For this review, take the finished solid that the model builds, in its own axes (mm). Face numbers are marked on the shaded views. A direction names the side the tool comes from. Round coordinates to 2 decimals unless told otherwise and drop trailing zeros. Order: outer loops, then holes, each group sorted by start corner. A loop starts at its lowest first (then second) coordinate and runs counter-clockwise, first axis right, second up. Notation, with made-up numbers: M 53.5,75 L 85.5,75 A28 cw 85.5,111 Z; hole C 76.25,66 d9. An arc over 180 degrees is marked long. Put each result on its own line as item: value.
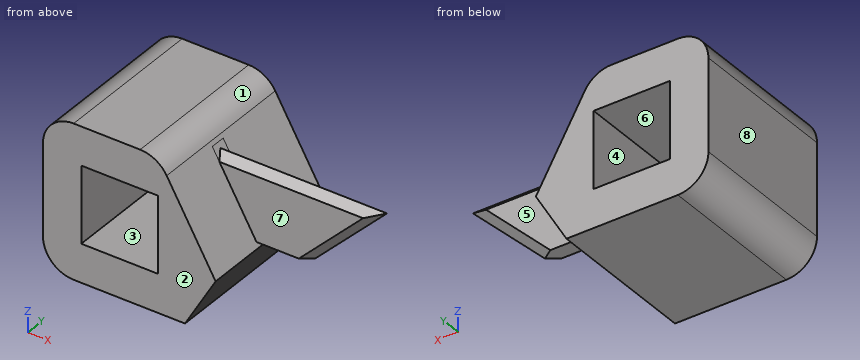
from build123d import *

# Parameters (mm, degrees)
F0_W        = 12.7
F0_H        = 12.7
F1_DEPTH    = 25.4
F4_DEPTH    = 2.54
F5_R        = 5.08
F6_SIZE     = 10.16
F7_T4_DEPTH = 40.3682325584
F7_T9_DEPTH = 40.3682325584
F8_T1_DEPTH = 25.5381499465


# Not quite as in the source:
# - a fillet or chamfer that OpenCascade refuses, or shapes differently, is made with other operations: its cross-section is extruded or revolved along the edge and cut away or added
# - a feature names something its author has since deleted; it is built from what else it names


with BuildPart() as f1:
    # F0 (on Front) → F1 (new body)
    with BuildSketch(Plane.XZ):
        Polygon((19.05, 25.4), (0, 25.4), (0, 0), (33.7146968374, 0), align=None)
        with Locations((12.7, 12.7)):
            Rectangle(F0_W, F0_H, mode=Mode.SUBTRACT)
    extrude(amount=F1_DEPTH)

    # F3 (on mid) → F4 (join)
    with BuildSketch(Plane.XZ.offset(12.7)):
        Polygon((50.8, 22.225), (20.8830871047, 22.225), (28.2154355234, 9.525), (38.1, 9.525), align=None)
    extrude(amount=F4_DEPTH)

    # F5
    f5_edges = [f1.edges().sort_by_distance(p)[0] for p in [
        (0, -12.7, 0),
        (0, -12.7, 25.4),
        (19.05, -12.7, 25.4),
    ]]
    fillet(f5_edges, radius=F5_R)

    # F6
    f6_edges = [f1.edges().sort_by_distance(p)[0] for p in [
        (33.714697, -12.7, 0),
    ]]
    chamfer(f6_edges, length=F6_SIZE)

    # F7: chamfer of 2.032 on 2 edges, made by hand


with BuildPart() as f7_tool2:
    # F7_s3 → F7_t4 (new body)
    with BuildSketch(Plane.YZ.offset(56.0256598315)):
        Polygon((-14.732, 22.225), (-12.7, 20.193), (-12.7, 22.225), align=None)
    extrude(amount=-F7_T4_DEPTH)

    split(bisect_by=Plane(origin=(25.2860226281, 0, 14.598891971), x_dir=(0, 1, 0), z_dir=(0.8660254038, 0, 0.5)), keep=Keep.TOP)


with BuildPart() as f1_1:
    add(f1.part)

    # F7_t1: cut F7_tool2
    add(f7_tool2.part, mode=Mode.SUBTRACT)


with BuildPart() as f7_tool7:
    # F7_s8 → F7_t9 (new body)
    with BuildSketch(Plane.YZ.offset(56.0256598315)):
        Polygon((-15.24, 20.193), (-13.208, 22.225), (-15.24, 22.225), align=None)
    extrude(amount=-F7_T9_DEPTH)

    split(bisect_by=Plane(origin=(25.2860226281, 0, 14.598891971), x_dir=(0, 1, 0), z_dir=(0.8660254038, 0, 0.5)), keep=Keep.TOP)


with BuildPart() as f1_2:
    add(f1_1.part)

    # F7_t6: cut F7_tool7
    add(f7_tool7.part, mode=Mode.SUBTRACT)

    # F8: chamfer of 2.032 on 2 edges, made by hand

    # F8_s2 → F8_t1 (cut)
    with BuildSketch(Plane(origin=(20.1174004969, 0, 20.1174004969), x_dir=(0, 1, 0), z_dir=(0.7071067812, 0, 0.7071067812))):
        Polygon((-12.7, -18.1735762724), (-14.732, -20.2055762724), (-12.7, -20.2055762724), align=None)
        Polygon((-15.24, -18.1735762724), (-13.208, -20.2055762724), (-15.24, -20.2055762724), align=None)
    extrude(amount=F8_T1_DEPTH, mode=Mode.SUBTRACT)


solid = f1_2.part
(1) Add section D-D on x = 32. Give the boundary of the cut face in (y, z) (3 decimals), then the cut area to 3 significant figures.
A:
outline: M -15.24,9.525 L -12.7,9.525 L -12.7,20.193 L -13.97,21.463 L -15.24,20.193 Z
area: 28.7 mm2
(2) To check wall thickness, follow L1, parallel to Z at x = 14, y = -15.5; L2, parallel to Y at x = 38.5, z = 13; L3, parallel to X at y = -10, z = 10.25. State the ranges of each line that lie inside material, in increasing order.
A:
L1: z = 0 to 6.35, 19.05 to 25.4
L2: y = -15.24 to -12.7
L3: x = 0 to 6.35, 19.05 to 27.8
(3) Add section A-A on x = 8. Give the boundary of the cut face in (y, z), then the cut area to 3 significant figures.
A:
outline: M -25.4,0 L 0,0 L 0,6.35 L -25.4,6.35 Z; M -25.4,19.05 L 0,19.05 L 0,25.4 L -25.4,25.4 Z
area: 323 mm2
(4) Add section C-C on z = 18. Give the boundary of the cut face in (x, y).
A:
outline: M 0,-25.4 L 6.35,-25.4 L 6.35,0 L 0,0 Z; M 19.05,-25.4 L 23.32,-25.4 L 23.32,-15.24 L 43.7,-15.24 L 45.5,-13.97 L 43.7,-12.7 L 23.32,-12.7 L 23.32,0 L 19.05,0 Z
(5) Insertion check: pin 1 Ø1 at (x, y) = (27.5, -5) entering from +Z; pin 2 Ø3 at (y, z) = (-19.5, 3) entering from -X; pin 3 Ø4 at (y, z) = (-11.5, 10) entering from +X; pin 4 Ø6 at (x, y) = (26, -19.5) entering from -Z. Each pin has a flat end and moves straight along its axis. Give the tip position at first contact, or say it passes through.
A:
pin 1: stops at z = 11.63
pin 2: stops at x = 0.03
pin 3: stops at x = 37.47
pin 4: stops at z = 0
(6) For the marked faces 5, 6, 7 and 8, list the 3-axis set-ups (+Z, -Z, +X, -X, +Y, -Y) from which the entire face can be reached by the end or side of a thin tool; tool diameter is ignored.
A:
face 5: +Z, +X, +Y
face 6: +Y, -Y
face 7: +Z, +X, -Y
face 8: +Z, -Z, -X, +Y, -Y
(7) Draft analysis for pull direction X (two halves, no side actions). For the marked faces 1, 2, 3 and 4, state which applies: released by +X, released by -X, zero draft, split by the parting line, or undercut.
A:
face 1: released by +X
face 2: zero draft
face 3: undercut
face 4: undercut
(8) Add section B-B on y = -23.5. Give the boundary of the cut face in (x, z).
A:
outline: M 0,5.08 A5.08 ccw 5.08,0 L 23.55,0 L 28.63,8.8 L 20.52,22.86 A5.08 ccw 16.12,25.4 L 5.08,25.4 A5.08 ccw 0,20.32 Z; hole M 6.35,6.35 L 19.05,6.35 L 19.05,19.05 L 6.35,19.05 Z
